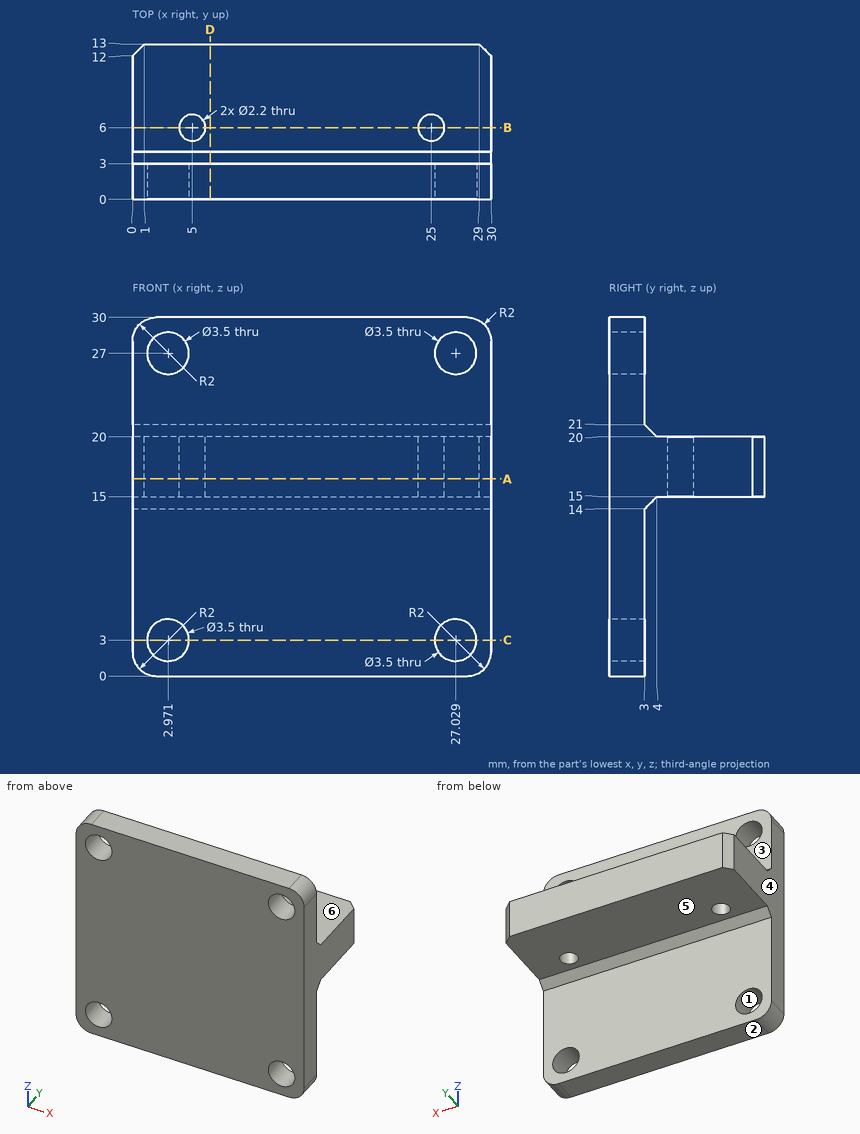
Study the drawing (mm; zero at the part's minimum x, y, z) and answer. A direction names the side the tool comes from. Coordinates: 2 decimals unless noted, no trailing zeros. Loops run counter-clockwise (first coordinate to the right, second up) from the corner with the lowest first, then second, coordinate; pieces in that order, holes last. Notation, with made-up numbers: (-26.5, 71.5) -> (-6.5, 71.5) arc R17 cw to (-6.5, 101.5) -> close; hole circle Ø6 at (14, -11). An arc over 180 degrees is marked (long way). Answer as CSV lines item,"result".
1) Straight lines are drawn through the part: probe 1 along X at (y, z) = (0.95, 3); probe 2 along Y at (x, z) = (5, 16.3); probe 3 along Y at (x, z) = (14.75, 2.25). For each, find the intervals that lie inside material, in ascending order.
A:
probe 1,"x = 0 to 1.22, 4.72 to 25.28, 28.78 to 30"
probe 2,"y = 0 to 4.9, 7.1 to 13"
probe 3,"y = 0 to 3"
2) For a pull along Z with two mould halves and no side action, classify the marked faces 1, 2 and 3 as released by +Z, released by -Z, zero draft, split by the parting line, or undercut.
A:
face 1,"undercut"
face 2,"released by -Z"
face 3,"zero draft"
3) The part is cut by section D-D (x = 6.5). Give the vertices of the cut face in (y, z).
A:
outline,"(0, 0) -> (3, 0) -> (3, 14) -> (4, 15) -> (13, 15) -> (13, 20) -> (4, 20) -> (3, 21) -> (3, 30) -> (0, 30) -> close"
4) The part is cut by section B-B (y = 6). Give the vertices of the cut face in (x, z).
A:
outline,"(0, 15) -> (3.9, 15) -> (3.9, 20) -> (0, 20) -> close; (6.1, 15) -> (23.9, 15) -> (23.9, 20) -> (6.1, 20) -> close; (26.1, 15) -> (30, 15) -> (30, 20) -> (26.1, 20) -> close"
5) The part is cut by section C-C (z = 3). Give the vertices of the cut face in (x, y).
A:
outline,"(0, 0) -> (1.22, 0) -> (1.22, 3) -> (0, 3) -> close; (4.72, 0) -> (25.28, 0) -> (25.28, 3) -> (4.72, 3) -> close; (28.78, 0) -> (30, 0) -> (30, 3) -> (28.78, 3) -> close"
6) The part is cut by section A-A (z = 16.5). Give the vertices of the cut face in (x, y), and give its area (3 significant figures).
A:
outline,"(0, 0) -> (30, 0) -> (30, 12) -> (29, 13) -> (1, 13) -> (0, 12) -> close; hole circle Ø2.2 at (5, 6); hole circle Ø2.2 at (25, 6)"
area,"381 mm²"
7) Flat-ended cylindrical pins translate along their axes: pin 1 (10 mm diameter, centred on x = 7, z = 27, fed in from -Y); pin 2 (4 mm diameter, centred on x = 2.97, z = 3, fed in from +Y); pin 3 (2.5 mm diameter, centred on x = 9.5, y = 7, fed in from -Z); pin 4 (2.5 mm diameter, centred on x = 16, y = 10.5, fed in from +Z). Find the tip coordinate at first contact, or state that the pin passes through.
A:
pin 1,"stops at y = 0"
pin 2,"stops at y = 3"
pin 3,"stops at z = 15"
pin 4,"stops at z = 20"
8) For the marked faces 4, 5 and 6, determine the directions among +Z, -Z, +X, -X, +Y, -Y from which every point of the face is accessible in a straight line to the end or side of a thin tool.
A:
face 4,"+Z, -Z, -X, +Y, -Y"
face 5,"-Z, +X, -X, +Y"
face 6,"+Z, +X, -X, +Y"
